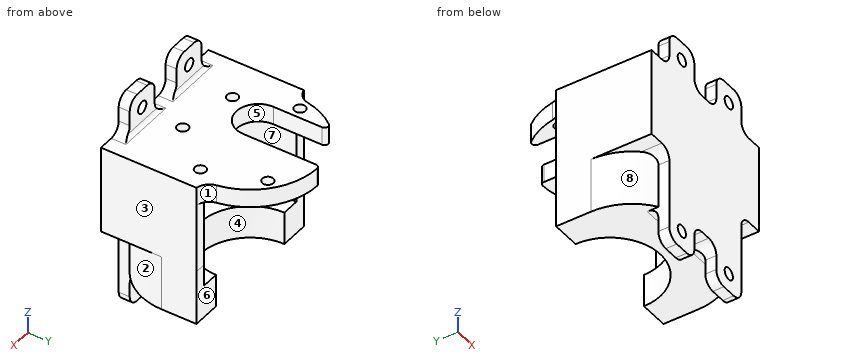
```python
from build123d import *

# Parameters (mm, degrees)
BOSS_EXTRUDE1_DEPTH      = 9
BOSS_EXTRUDE2_DEPTH      = 25
FILLET1_R                = 16.5
BOSS_EXTRUDE3_START      = -34
SKETCH4_W                = 10
SKETCH4_H                = 3
BOSS_EXTRUDE3_DEPTH      = 44
SKETCH5_R                = 1.65
CUT_EXTRUDE1_DEPTH       = 3
FILLET2_R                = 3
SKETCH12_R               = 18.5
SKETCH12_R_2             = 1.5
SKETCH12_R_3             = 6
BOSS_EXTRUDE8_DEPTH      = 5
BOSS_EXTRUDE9_DEPTH      = 5
BOSS_EXTRUDE9_DEPTH_BACK = 19
SKETCH14_R               = 1.65
BOSS_EXTRUDE11_DEPTH     = 3
CUT_EXTRUDE2_START       = -6
CUT_EXTRUDE2_DEPTH       = 6
FILLET4_R                = 1
FILLET5_START            = -13
FILLET5_DEPTH            = 6
FILLET5_2_DEPTH          = 4
FILLET5_START_2          = -18
FILLET5_3_DEPTH          = 36
FILLET6_R                = 4


with BuildPart() as part:
    # Sketch1 → Boss-Extrude1 (new body)
    with BuildSketch(Plane.XY):
        with BuildLine():
            Line((13.7, 13), (21.5, 13))
            Line((21.5, 13), (21.5, -13))
            Line((21.5, -13), (-21.5, -13))
            Line((-21.5, -13), (-21.5, 13))
            Line((-21.5, 13), (-13.7, 13))
            ThreePointArc((-13.7, 13), (0, -0.7), (13.7, 13))
        make_face()
    extrude(amount=BOSS_EXTRUDE1_DEPTH)

    # Sketch2 → Boss-Extrude2 (add)
    with BuildSketch(Plane.XY.offset(9)):
        with BuildLine():
            Line((18.5, 13), (21.5, 13))
            Line((21.5, 13), (21.5, -13))
            Line((21.5, -13), (-21.5, -13))
            Line((-21.5, -13), (-21.5, 13))
            Line((-21.5, 13), (-18.5, 13))
            ThreePointArc((-18.5, 13), (0, -5.5), (18.5, 13))
        make_face()
    extrude(amount=BOSS_EXTRUDE2_DEPTH)

    # Fillet1
    fillet1_edges = [part.edges().sort_by_distance(p)[0] for p in [
        (21.5, -13, 17),
        (-21.5, -13, 17),
    ]]
    fillet(fillet1_edges, radius=FILLET1_R)

    # Sketch4 → Boss-Extrude3 (add)
    with BuildSketch(Plane(origin=(0, 0, 0), x_dir=(-1, 0, 0), z_dir=(0, 0, -1)).offset(BOSS_EXTRUDE3_START)):
        with Locations((-9.4, -11.5)):
            Rectangle(SKETCH4_W, SKETCH4_H)
        with Locations((9.4, -11.5)):
            Rectangle(SKETCH4_W, SKETCH4_H)
    extrude(amount=BOSS_EXTRUDE3_DEPTH)

    # Sketch5 → Cut-Extrude1 (cut)
    with BuildSketch(Plane(origin=(0, -10, 0), x_dir=(1, 0, 0), z_dir=(0, 1, 0))):
        with Locations(Location((9.4, 5, 0), (0, 0, 180))):
            Circle(SKETCH5_R)
        with Locations(Location((-9.4, 5, 0), (0, 0, 270))):
            Circle(SKETCH5_R)
    extrude(amount=-CUT_EXTRUDE1_DEPTH, mode=Mode.SUBTRACT)

    # Fillet2
    fillet2_edges = [part.edges().sort_by_distance(p)[0] for p in [
        (4.4, -11.5, 0),
        (9.4, -10, 0),
        (14.4, -11.5, -10),
        (4.4, -11.5, -10),
        (-9.4, -10, 0),
        (-4.4, -11.5, 0),
        (-14.4, -11.5, -10),
        (-4.4, -11.5, -10),
    ]]
    fillet(fillet2_edges, radius=FILLET2_R)



with BuildPart() as body_2:
    # Sketch12 → Boss-Extrude8 (new body)
    with BuildSketch(Plane.XY.offset(34)):
        with Locations((0, 13)):
            Circle(SKETCH12_R)
        with Locations((-15.451860729, 16.05)):
            Circle(SKETCH12_R_2, mode=Mode.SUBTRACT)
        with Locations((-5.084552883, 27.906703927)):
            Circle(SKETCH12_R_2, mode=Mode.SUBTRACT)
        with Locations((10.367307846, 24.856703927)):
            Circle(SKETCH12_R_2, mode=Mode.SUBTRACT)
        with Locations((15.451860729, 9.95)):
            Circle(SKETCH12_R_2, mode=Mode.SUBTRACT)
        with Locations((5.084552883, -1.906703927)):
            Circle(SKETCH12_R_2, mode=Mode.SUBTRACT)
        with Locations((-10.367307846, 1.143296073)):
            Circle(SKETCH12_R_2, mode=Mode.SUBTRACT)
        with Locations((-6.625133961, 10.74)):
            Circle(SKETCH12_R_3, mode=Mode.SUBTRACT)
    extrude(amount=BOSS_EXTRUDE8_DEPTH)


with BuildPart() as part_1:
    add(part.part)

    add(body_2.part)  # Boss-Extrude9 merges body 2
    # Sketch13 → Boss-Extrude9 (add, two sides: drawn at the far end of the back side and taken through both)
    with BuildSketch(Plane.XY.offset(34).offset(-BOSS_EXTRUDE9_DEPTH_BACK)):
        with BuildLine():
            Line((-21.5, 13), (-21.5, -13))
            Line((-21.5, -13), (21.5, -13))
            Line((21.5, -13), (21.5, 13))
            Line((21.5, 13), (18.496156013, 13.034404843))
            Line((18.496156013, 13.034404843), (18.5, 13))
            ThreePointArc((18.5, 13), (0, -5.5), (-18.5, 13))
            Line((-18.5, 13), (-21.5, 13))
        make_face()
    extrude(amount=BOSS_EXTRUDE9_DEPTH + BOSS_EXTRUDE9_DEPTH_BACK)

    # Sketch14 → Boss-Extrude11 (add)
    # profile 1 of 2: a face of its own
    with BuildSketch(Plane.XZ.offset(13)):
        with BuildLine():
            Line((7.4, 49), (11.4, 49))
            ThreePointArc((11.4, 49), (13.521320344, 48.121320344), (14.4, 46))
            Line((14.4, 46), (14.4, 39))
            Line((14.4, 39), (4.4, 39))
            Line((4.4, 39), (4.4, 46))
            ThreePointArc((4.4, 46), (5.278679656, 48.121320344), (7.4, 49))
        make_face()
        with Locations(Location((9.4, 44, 0), (0, 0, 180))):
            Circle(SKETCH14_R, mode=Mode.SUBTRACT)
    # profile 2 of 2: a face of its own
    with BuildSketch(Plane.XZ.offset(13)):
        with BuildLine():
            Line((-7.4, 49), (-11.4, 49))
            ThreePointArc((-11.4, 49), (-13.521320344, 48.121320344), (-14.4, 46))
            Line((-14.4, 46), (-14.4, 39))
            Line((-14.4, 39), (-4.4, 39))
            Line((-4.4, 39), (-4.4, 46))
            ThreePointArc((-4.4, 46), (-5.278679656, 48.121320344), (-7.4, 49))
        make_face()
        with Locations(Location((-9.4, 44, 0), (0, 0, 180))):
            Circle(SKETCH14_R, mode=Mode.SUBTRACT)
    extrude(amount=-BOSS_EXTRUDE11_DEPTH)

    # Sketch15 → Cut-Extrude2 (cut)
    with BuildSketch(Plane.XY.offset(39).offset(CUT_EXTRUDE2_START)):
        with BuildLine():
            Line((-12.625133961, 10.74), (-12.625133961, 26.522425539))
            ThreePointArc((-12.625133961, 26.522425539), (-7.075323018, 30.093560314), (-0.625133961, 31.489435025))
            Line((-0.625133961, 31.489435025), (-0.625133961, 10.74))
            ThreePointArc((-0.625133961, 10.74), (-6.625133961, 4.74), (-12.625133961, 10.74))
        make_face()
    extrude(amount=CUT_EXTRUDE2_DEPTH, mode=Mode.SUBTRACT)

    # Fillet4
    fillet4_edges = [part_1.edges().sort_by_distance(p)[0] for p in [
        (-9.4, -10, 39),
        (9.4, -10, 39),
        (-12.625133961, 26.522425539, 36.5),
        (-0.625133961, 31.489435025, 36.5),
    ]]
    fillet(fillet4_edges, radius=FILLET4_R)

    # Fillet5: read off the stored shape, not the designer's step
    # Fillet5 outline → Fillet5 (add)
    with BuildSketch(Plane(origin=(0, 0, 0), x_dir=(1, 0, 0), z_dir=(0, 1, 0)).offset(FILLET5_START)):
        with BuildLine():
            ThreePointArc((-14.4, -12), (-15.278679656, -14.121320344), (-17.4, -15))
            Line((-17.4, -15), (-14.4, -15))
            Line((-14.4, -15), (-14.4, -12))
        make_face()
        with BuildLine():
            Line((14.4, -15), (17.4, -15))
            ThreePointArc((17.4, -15), (15.278679656, -14.121320344), (14.4, -12))
            Line((14.4, -12), (14.4, -15))
        make_face()
    extrude(amount=FILLET5_DEPTH)

    # Fillet5 2 outline → Fillet5 2 (add)
    with BuildSketch(Plane(origin=(0, 0, 0), x_dir=(1, 0, 0), z_dir=(0, 1, 0)).offset(FILLET5_START)):
        with BuildLine():
            Line((14.4, -39), (14.4, -42))
            ThreePointArc((14.4, -42), (15.278679656, -39.878679656), (17.4, -39))
            Line((17.4, -39), (14.4, -39))
        make_face()
        with BuildLine():
            Line((-14.4, -42), (-14.4, -39))
            Line((-14.4, -39), (-17.4, -39))
            ThreePointArc((-17.4, -39), (-15.278679656, -39.878679656), (-14.4, -42))
        make_face()
        with BuildLine():
            ThreePointArc((-4.4, -42), (-3.521320344, -39.878679656), (-1.4, -39))
            Line((-1.4, -39), (-4.4, -39))
            Line((-4.4, -39), (-4.4, -42))
        make_face()
        with BuildLine():
            Line((4.4, -42), (4.4, -39))
            Line((4.4, -39), (1.4, -39))
            ThreePointArc((1.4, -39), (3.521320344, -39.878679656), (4.4, -42))
        make_face()
    extrude(amount=FILLET5_2_DEPTH)

    # Fillet5 3 outline → Fillet5 3 (cut)
    with BuildSketch(Plane.YZ.offset(FILLET5_START_2)):
        with BuildLine():
            Line((-9, 42), (-10, 42))
            Line((-10, 42), (-10, 40))
            ThreePointArc((-10, 40), (-9.707106781, 39.292893219), (-9, 39))
            Line((-9, 39), (-9, 42))
        make_face()
    extrude(amount=FILLET5_3_DEPTH, mode=Mode.SUBTRACT)

    # Fillet6
    # the kernel refuses this fillet: 4 mm, written as the material it adds along each edge
    with BuildSketch(Plane(origin=(-18.5, 13, 39), x_dir=(-1, 0, 0), z_dir=(0, 0, -1))) as fillet6_piece_1:
        with BuildLine():
            CenterArc((3.651162791, 3.9466425), FILLET6_R, 190.102305056, 70.528779366)
            ThreePointArc((-0.286821705, 3.245017166), (-0.071844932, 1.628834177), (0, 0))
            Line((0, 0), (3, 0))
        make_face()
    extrude(amount=5)
    with BuildSketch(Plane(origin=(18.499968089, 13.034361181, 39), x_dir=(-0.08897012709688518, 0.996034294833448, 0), z_dir=(0, 0, -1))) as fillet6_piece_2:
        with BuildLine():
            CenterArc((3.571919108, 3.984791306), FILLET6_R, 194.473277614, 70.528779366)
            Line((-0.301138135, 2.98507755), (0, 0))
            ThreePointArc((0, 0), (1.611719597, 0.070340211), (3.223439195, 0))
        make_face()
    extrude(amount=5)


solid = part_1.part
```
The listing builds one solid part. Answer for the finished solid, in the listing's coordinates (mm). Face numbers are marked on the shaded views. A direction names the side the tool comes from. Give positions to 0.01 mm unless a question says otherwise; leave off trailing zeros. Order: outer loops, then holes, each group sorted by start corner. A loop starts at its lowest first (then second) coordinate and runs counter-clockwise, first axis right, second up. Notation, with made-up numbers: (12, 21) -> (27, 21) arc R25 ccw to (27, 42) -> close; hole circle Ø6 at (68.5, -39). An arc over 180 degrees is marked (long way). Answer as a JSON object with one key per item and string values. Group by question number.
Item 1: A tool of negligible diameter and unlimited length cuts with its end or side. For the marked faces 1, 2, 3 and 4, from which of +Z, -Z, +X, -X, +Y, -Y can it reach the whole face along a straight path? Write none if from no direction.
Item 2: Flat-ended cylindrical pins translate along their axes: pin 1 (0.9 mm diameter, centred on y = -11, z = 45, fed in from +X); pin 2 (3 mm diameter, centred on x = 9.4, z = 44, fed in from +Y); pin 3 (5 mm diameter, centred on x = 5.08, y = -1.91, fed in from +Z); pin 4 (7.5 mm diameter, centred on x = -11, z = -8, fed in from +Y). Find the tip coordinate at first contact, or state that the pin passes through.
Item 3: The part is cut by section A-A on z = 44. Write down the section's boundary in (x, y).
Item 4: The part is cut by section B-B on y = 9.95. Write down the section's boundary in (x, z).
Item 5: Consider L1, parallel to X at y = -11.65, z = 44; L2, parallel to Z at x = -9, y = -11; L3, parallel to X at y = 16, z = 37. Determine where each line is inside the solid, lowest interval first. Write a range as from..to.
Item 6: Determine the mould class of the marked faces 5, 6, 7 and 8 for opening direction X: pulls with the +X half, pulls with the -X half, needs draft (parallel to the pull), parting line crosses it, or undercut.
Item 7: The part is cut by section C-C on y = 21. Write down the section's boundary in (x, z), and give its area (3 significant figures).
Result set:
{
 "1": {"face 1": "+Z, -Z, +X, +Y", "face 2": "-Z, +X, -Y", "face 3": "+Z, -Z, +X, +Y, -Y", "face 4": "-Z, +Y"},
 "2": {"pin 1": "x = 14.4", "pin 2": "through", "pin 3": "z = 39", "pin 4": "y = -10"},
 "3": {"outline": "(-14.4, -13) -> (-11.05, -13) -> (-11.05, -10) -> (-14.4, -10) -> close; (-7.75, -13) -> (-4.4, -13) -> (-4.4, -10) -> (-7.75, -10) -> close; (4.4, -13) -> (7.75, -13) -> (7.75, -10) -> (4.4, -10) -> close; (11.05, -13) -> (14.4, -13) -> (14.4, -10) -> (11.05, -10) -> close"},
 "4": {"outline": "(-21.5, 0) -> (-13.36, 0) -> (-13.36, 9) -> (-18.25, 9) -> (-18.25, 34) -> (-12.57, 34) -> (-12.57, 39) -> (-21.5, 39) -> close; (-0.68, 34) -> (13.95, 34) -> (13.95, 39) -> (-0.68, 39) -> close; (13.36, 0) -> (21.5, 0) -> (21.5, 39) -> (16.95, 39) -> (16.95, 34) -> (18.25, 34) -> (18.25, 9) -> (13.36, 9) -> close"},
 "5": {"L1": "-14.4..-11.05, -7.75..-4.4, 4.4..7.75, 11.05..14.4", "L2": "-10..-6.6, -3.4..42.4, 45.6..49", "L3": "-18.26..-16.95, -13.95..-12.63, -0.63..18.26"},
 "6": {"face 5": "undercut", "face 6": "needs draft", "face 7": "undercut", "face 8": "pulls with the -X half"},
 "7": {"outline": "(-16.68, 34) -> (-12.63, 34) -> (-12.63, 39) -> (-16.68, 39) -> close; (-0.63, 34) -> (16.68, 34) -> (16.68, 39) -> (-0.63, 39) -> close", "area": "107 mm²"}
}
